```python
from build123d import *

# Parameters (mm, degrees)
F0_W     = 203.2
F0_H     = 127
F1_DEPTH = 127
F3_DEPTH = 76.2
F4_SIZE2 = 101.6
F4_SIZE  = 76.2
F5_R     = 5.08
F6_R     = 15.24
F7_DEPTH = 50.8
F8_R     = 17.3644725526
F9_DEPTH = 127


with BuildPart() as f1:
    # F0 (on Front) → F1 (new body)
    with BuildSketch(Plane.XZ):
        Rectangle(F0_W, F0_H)
    extrude(amount=F1_DEPTH)

    # F2 (on face) → F3 (cut)
    with BuildSketch(Plane.XZ.offset(127)):
        Polygon((101.6, 63.5), (0, 63.5), (0, 0), (-49.4145452976, 0), (-49.4145452976, -63.5), (101.6, -63.5), align=None)
    extrude(amount=-F3_DEPTH, mode=Mode.SUBTRACT)

    # F4
    f4_edges = [f1.edges().sort_by_distance(p)[0] for p in [
        (101.6, -25.4, 63.5),
    ]]
    f4_side = f1.faces().sort_by_distance((-21.771429, -52.614286, 63.5))[0]
    chamfer(f4_edges, length=F4_SIZE, length2=F4_SIZE2, reference=f4_side)

    # F5
    f5_edges = [f1.edges().sort_by_distance(p)[0] for p in [
        (25.4, -25.4, 63.5),
        (12.7, -50.8, 63.5),
        (0, -88.9, 63.5),
        (-50.8, -127, 63.5),
        (-101.6, -63.5, 63.5),
        (-38.1, 0, 63.5),
        (-101.6, -127, 0),
        (-49.414545, -127, -31.75),
        (-24.707273, -127, 0),
        (0, -88.9, 0),
        (0, -127, 31.75),
        (-75.507273, -127, -63.5),
        (0, -50.8, 31.75),
        (-101.6, 0, 0),
        (-101.6, -63.5, -63.5),
        (0, 0, -63.5),
        (26.092727, -50.8, -63.5),
        (-49.414545, -88.9, -63.5),
        (-49.414545, -50.8, -31.75),
        (-24.707273, -50.8, 0),
    ]]
    fillet(f5_edges, radius=F5_R)

    # F6 (on face) → F7 (cut, through all)
    with BuildSketch(Plane.XZ.offset(50.8)):
        with Locations((6.4654547024, -17.78)):
            Circle(F6_R)
    extrude(amount=-F7_DEPTH, mode=Mode.SUBTRACT)

    # F8 (on face) → F9 (cut, through all)
    with BuildSketch(Plane.XY.offset(63.5)):
        with Locations((-58.8048510253, -64.9624243379)):
            Circle(F8_R)
    extrude(amount=-F9_DEPTH, mode=Mode.SUBTRACT)


solid = f1.part
```
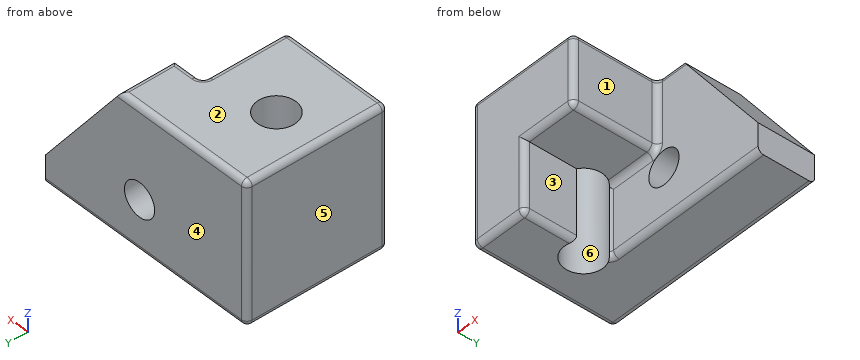
Verification items for the finished model (mm, model axes). Face numbers are marked on the shaded views. A direction names the side the tool comes from. Give positions to 0.01 mm unless a question says otherwise; leave off trailing zeros. Order: outer loops, then holes, each group sorted by start corner. A loop starts at its lowest first (then second) coordinate and runs counter-clockwise, first axis right, second up. Notation, with made-up numbers: (-28.5, 70) -> (12.5, 70) arc R12 cw to (12.5, 86) -> close; hole circle Ø1 at (31, 8). An arc over 180 degrees is marked (long way). One line per item, written item: value.
(1) Sectioned sample at A-A on z = -17.78. Record the cut outline in (x, y).
Final values:
outline: (-101.6, -121.92) arc R5.08 ccw to (-96.52, -127) -> (-54.49, -127) arc R5.08 ccw to (-49.41, -121.92) -> (-49.41, -79.57) arc R17.36 cw (long way) to (-47.42, -51.85) arc R5.08 cw to (-44.33, -50.8) -> (-8.77, -50.8) -> (-8.77, 0) -> (-96.52, 0) arc R5.08 ccw to (-101.6, -5.08) -> close; (21.71, -50.8) -> (86.36, -50.8) -> (86.36, 0) -> (21.71, 0) -> close
(2) Draft check along X on the marked faces 4, 5 and 6. Enter one of: pulls with the +X half, pulls with the -X half, needs draft (parallel to the pull), parting line crosses it, or undercut.
Final values:
face 4: needs draft
face 5: pulls with the -X half
face 6: undercut
(3) Tool access check on the marked faces 1, 2 and 3. Record the directions out of +Z, -Z, +X, -X, +Y, -Y that give a thin tool (end or side, any length) a straight path to the whole face; none if there is none.
Final values:
face 1: +Z, -Z, +X, -Y
face 2: +Z, +X, -X, +Y, -Y
face 3: -Z, +X, -Y
(4) Sectioned sample at C-C on z = 23.5. Record the cut outline in (x, y), then the cut area to 3 significant figures.
Final values:
outline: (-101.6, -121.92) arc R5.08 ccw to (-96.52, -127) -> (-5.08, -127) arc R5.08 ccw to (0, -121.92) -> (0, -55.88) arc R5.08 cw to (5.08, -50.8) -> (55.4, -50.8) -> (55.4, 0) -> (-96.52, 0) arc R5.08 ccw to (-101.6, -5.08) -> close; hole circle Ø34.73 at (-58.8, -64.96)
area: 14,800 mm^2
(5) Scan lines: line 1 along Z through (x, y) = (6, -40); line 2 along Y through (x, z) = (-73, -15); line 3 along Y through (x, z) = (11, 24). Record each from-to range of solid material in increasing order. Write a range as [from, to].
Final values:
line 1: [-63.5, -33.01], [-2.55, 63.5]
line 2: [-127, -74.96], [-54.96, 0]
line 3: [-50.8, 0]
(6) Sectioned sample at B-B on y = -98. Record the cut outline in (x, z), then the cut area to 3 significant figures.
Final values:
outline: (-101.6, -58.42) arc R5.08 ccw to (-96.52, -63.5) -> (-54.49, -63.5) arc R5.08 ccw to (-49.41, -58.42) -> (-49.41, 0) -> (-5.08, 0) arc R5.08 ccw to (0, 5.08) -> (0, 58.42) arc R5.08 ccw to (-5.08, 63.5) -> (-96.52, 63.5) arc R5.08 ccw to (-101.6, 58.42) -> close
area: 9,740 mm^2
(7) Gauge pin test, flat ends, axial feed: pin 1 (1 mm diameter, centred on x = -3.5, y = -111.5, fed in from +Z); pin 2 (4 mm diameter, centred on x = -19, y = -103, fed in from -Z); pin 3 (5 mm diameter, centred on y = -57, z = 43, fed in from +X). Record the tip position at first contact, or that the pin passes through.
Final values:
pin 1: z = 63.38
pin 2: z = 0
pin 3: x = 0.19
(8) Sectioned sample at D-D on y = -76. Record the cut outline in (x, z).
Final values:
outline: (-101.6, -58.42) arc R5.08 ccw to (-96.52, -63.5) -> (-72.21, -63.5) -> (-72.21, 63.5) -> (-96.52, 63.5) arc R5.08 ccw to (-101.6, 58.42) -> close; (-45.4, 0) -> (-5.08, 0) arc R5.08 ccw to (0, 5.08) -> (0, 58.42) arc R5.08 ccw to (-5.08, 63.5) -> (-45.4, 63.5) -> close
